```python
from build123d import *

# Parameters (mm, degrees)
F1_DEPTH = 609.6
F2_W     = 25.4
F2_H     = 101.6
F2_H_2   = 114.3
F3_DEPTH = 609.6
F4_W     = 152.4
F4_H     = 25.4
F4_W_2   = 25.4
F5_DEPTH = 2032


with BuildPart() as f1:
    # F0 (on Top) → F1 (new body)
    with BuildSketch(Plane.XY):
        Polygon((304.8, 812.8), (0, 812.8), (0, 0), (812.8, 0), (812.8, 25.4), (25.4, 25.4), (25.4, 787.4), (304.8, 787.4), align=None)
    extrude(amount=-F1_DEPTH)

    # F2 (on face) → F3 (join)
    with BuildSketch(Plane.XY):
        with Locations((292.1, 863.6)):
            Rectangle(F2_W, F2_H)
        with Locations((12.7, 869.95)):
            Rectangle(F2_W, F2_H_2)
    extrude(amount=-F3_DEPTH)

    # F4 (on Front) → F5 (cut)
    with BuildSketch(Plane.XZ):
        with Locations((101.6, -12.7)):
            Rectangle(F4_W, F4_H)
        with Locations((292.1, -12.7)):
            Rectangle(F4_W_2, F4_H)
        with Locations((101.6, -596.9)):
            Rectangle(F4_W, F4_H)
        with Locations((292.1, -596.9)):
            Rectangle(F4_W_2, F4_H)
    extrude(amount=-F5_DEPTH, mode=Mode.SUBTRACT)


solid = f1.part
```
Source: CAD feature listing. Evaluate the final solid. Frame: model axes, mm. A direction names the side the tool comes from. Round coordinates to 2 decimals unless told otherwise and drop trailing zeros. Order: outer loops, then holes, each group sorted by start corner. A loop starts at its lowest first (then second) coordinate and runs counter-clockwise, first axis right, second up. Notation, with made-up numbers: (22.25, -21.5) -> (60.25, -21.5) arc R28 cw to (60.25, 5.5) -> close; hole circle Ø11 at (71, 20). An arc over 180 degrees is marked (long way). One line per item, written item: value. Start each with the question number.
Q1. Pin query (flat end, axial travel): pin 1 (20.5 mm diameter, centred on x = 65, y = 17.5, fed in from +Z); pin 2 (1.5 mm diameter, centred on y = 559.5, z = -384, fed in from +X); pin 3 (8 mm diameter, centred on x = 315, z = -499, fed in from +Y). Return the tip coordinate at first contact, or that it passes through.
Q2. Section query A-A (x = 207). Return the cut outline in (y, z).
Q3. Access query for faces 4 (the flat face through (292, 850, -25.4)), 5 (the flat face through (101, 13, -584.2)), 6 (the flat face through (279.4, 800, -597)). Directions: +Z, -Z, +X, -X, +Y, -Y. A direction counts if a zero-diameter tool reaches every point of the face in a straight line with its end or side. Return the directions, or none.
Q4. Section query B-B (z = -466). Return the cut outline in (x, y).
Q5. Material intervals for probe 1 along X at (y, z) = (867.5, -281.5); probe 2 along Y at (x, z) = (212, -436.5); probe 3 along Y at (x, z) = (574, -135), sorted ascending.
Q6. Section query C-C (y = 497.5). Return the cut outline in (x, z).
Q7. Draft query along Y for faces 1 (the flat face through (425, 25.4, -301)), 2 (the flat face through (154, 812.8, -301)), 3 (the flat face through (812.8, 13, -301)). Return one class per face: pulls with the +Y half, pulls with the -Y half, needs draft (parallel to the pull), parting line crosses it, or undercut.
Findings below:
1. pin 1: z = -25.4
1. pin 2: x = 25.4
1. pin 3: y = 25.4
2. outline: (0, -609.6) -> (25.4, -609.6) -> (25.4, 0) -> (0, 0) -> close; (787.4, -609.6) -> (812.8, -609.6) -> (812.8, 0) -> (787.4, 0) -> close
3. face 4: +Z, +X, +Y, -Y
3. face 5: -Z, +Y, -Y
3. face 6: -Z, +X, +Y, -Y
4. outline: (0, 0) -> (812.8, 0) -> (812.8, 25.4) -> (25.4, 25.4) -> (25.4, 787.4) -> (304.8, 787.4) -> (304.8, 914.4) -> (279.4, 914.4) -> (279.4, 812.8) -> (25.4, 812.8) -> (25.4, 927.1) -> (0, 927.1) -> close
5. probe 1: 0 to 25.4, 279.4 to 304.8
5. probe 2: 0 to 25.4, 787.4 to 812.8
5. probe 3: 0 to 25.4
6. outline: (0, -609.6) -> (25.4, -609.6) -> (25.4, 0) -> (0, 0) -> close
7. face 1: undercut
7. face 2: pulls with the +Y half
7. face 3: needs draft
